from build123d import *

# Parameters (mm, degrees)
SKETCH1_W           = 25.4
SKETCH1_H           = 25.4
BOSS_EXTRUDE1_DEPTH = 228.6
FILLET1_R           = 1.5875
HOLE1_OUTLINE_R     = 2.5527
HOLE1_DEPTH         = 228.6
SKETCH7_W           = 6.5278
SKETCH7_H           = 2.2352
CUT_EXTRUDE2_DEPTH  = 228.6
FILLET4_R           = 0.396875
CIRPATTERN2_DEPTH   = 228.6


# Read off the part's stored shape, not the designer's step: Hole1, CirPattern2
with BuildPart() as part:
    # Sketch1 → Boss-Extrude1 (new body)
    with BuildSketch(Plane.XY):
        Rectangle(SKETCH1_W, SKETCH1_H)
    extrude(amount=BOSS_EXTRUDE1_DEPTH)

    # Fillet1
    fillet1_edges = [part.edges().sort_by_distance(p)[0] for p in [
        (12.7, -12.7, 114.3),
        (-12.7, -12.7, 114.3),
        (-12.7, 12.7, 114.3),
        (12.7, 12.7, 114.3),
    ]]
    fillet(fillet1_edges, radius=FILLET1_R)

    # Hole1 outline → Hole1 (cut)
    with BuildSketch(Plane.XY):
        with Locations((0, -0.048792482)):
            Circle(HOLE1_OUTLINE_R)
    extrude(amount=HOLE1_DEPTH, mode=Mode.SUBTRACT)

    # Sketch7 → Cut-Extrude2 (cut)
    with BuildSketch(Plane.XY.offset(228.6)):
        with Locations((0, 11.5824)):
            Rectangle(SKETCH7_W, SKETCH7_H)
        Polygon((-3.175, 4.5212), (-7.3025, 10.4648), (7.3025, 10.4648), (3.175, 4.5212), align=None)
    extrude(amount=-CUT_EXTRUDE2_DEPTH, mode=Mode.SUBTRACT)

    # Fillet4
    fillet4_edges = [part.edges().sort_by_distance(p)[0] for p in [
        (-3.2639, 10.4648, 114.3),
        (-3.2639, 12.7, 114.3),
        (3.2639, 12.7, 114.3),
        (3.2639, 10.4648, 114.3),
    ]]
    fillet(fillet4_edges, radius=FILLET4_R)

    # CirPattern2 outline → CirPattern2 (cut)
    with BuildSketch(Plane.XY):
        with BuildLine():
            ThreePointArc((-3.660775, -10.562384964), (-3.380141996, -10.67862696), (-3.2639, -10.959259964))
            Line((-3.2639, -10.959259964), (-3.2639, -12.7))
            Line((-3.2639, -12.7), (3.2639, -12.7))
            Line((3.2639, -12.7), (3.2639, -10.959259964))
            ThreePointArc((3.2639, -10.959259964), (3.380141996, -10.67862696), (3.660775, -10.562384964))
            Line((3.660775, -10.562384964), (7.3025, -10.562384964))
            Line((7.3025, -10.562384964), (3.175, -4.618784964))
            Line((3.175, -4.618784964), (-3.175, -4.618784964))
            Line((-3.175, -4.618784964), (-7.3025, -10.562384964))
            Line((-7.3025, -10.562384964), (-3.660775, -10.562384964))
        make_face()
        with BuildLine():
            Line((-12.7, -3.312692482), (-10.910467482, -3.312692482))
            ThreePointArc((-10.910467482, -3.312692482), (-10.629834478, -3.428934478), (-10.513592482, -3.709567482))
            Line((-10.513592482, -3.709567482), (-10.513592482, -7.351292482))
            Line((-10.513592482, -7.351292482), (-4.569992482, -3.223792482))
            Line((-4.569992482, -3.223792482), (-4.569992482, 3.126207518))
            Line((-4.569992482, 3.126207518), (-10.513592482, 7.253707518))
            Line((-10.513592482, 7.253707518), (-10.513592482, 3.611982518))
            ThreePointArc((-10.513592482, 3.611982518), (-10.629834478, 3.331349514), (-10.910467482, 3.215107518))
            Line((-10.910467482, 3.215107518), (-12.7, 3.215107518))
            Line((-12.7, 3.215107518), (-12.7, -3.312692482))
        make_face()
        with BuildLine():
            ThreePointArc((10.513592482, -3.709567482), (10.629834478, -3.428934478), (10.910467482, -3.312692482))
            Line((10.910467482, -3.312692482), (12.7, -3.312692482))
            Line((12.7, -3.312692482), (12.7, 3.215107518))
            Line((12.7, 3.215107518), (10.910467482, 3.215107518))
            ThreePointArc((10.910467482, 3.215107518), (10.629834478, 3.331349514), (10.513592482, 3.611982518))
            Line((10.513592482, 3.611982518), (10.513592482, 7.253707518))
            Line((10.513592482, 7.253707518), (4.569992482, 3.126207518))
            Line((4.569992482, 3.126207518), (4.569992482, -3.223792482))
            Line((4.569992482, -3.223792482), (10.513592482, -7.351292482))
            Line((10.513592482, -7.351292482), (10.513592482, -3.709567482))
        make_face()
    extrude(amount=CIRPATTERN2_DEPTH, mode=Mode.SUBTRACT)


solid = part.part
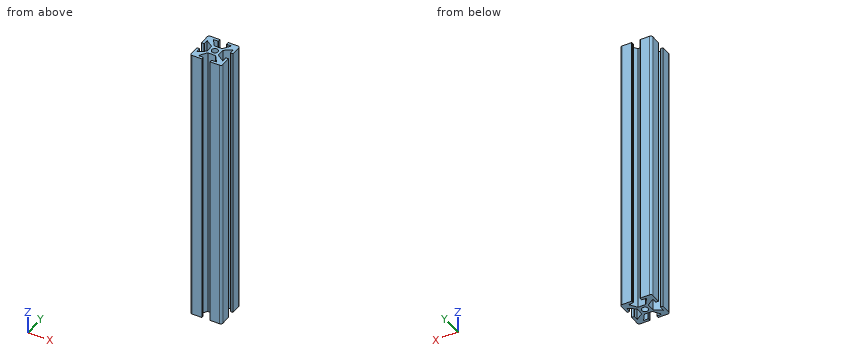
Work out the finished part from the listing and answer in its coordinate system (mm). Give positions to 0.01 mm unless a question says otherwise; leave off trailing zeros. Write each loop counter-clockwise with the first axis right and the second up, starting at its lowest first coordinate (ties: lowest second). Pieces come first, ordered by that corner, then holes.
Q1. Straight lines are drawn through the part: L1, parallel to Y at x = 11, z = 174; L2, parallel to Y at x = 0, z = 49.5; L3, parallel to X at y = 0, z = 47.5. For each, find the intervals that lie inside material, in ascending order.
Answer:
L1: y = -12.7 to -3.31, 3.22 to 12.7
L2: y = -4.62 to -2.6, 2.5 to 4.52
L3: x = -4.57 to -2.55, 2.55 to 4.57
Q2. The part is cut by section A-A on x = 0. Give the vertices of the cut face in (y, z).
Answer:
outline: (-4.62, 0) - (-2.6, 0) - (-2.6, 228.6) - (-4.62, 228.6) - close; (2.5, 0) - (4.52, 0) - (4.52, 228.6) - (2.5, 228.6) - close
Q3. Given pin 1 (0.5 mm diameter, centred on x = -11.5, z = 122.5, fed in from -Y); pin 2 (2 mm diameter, centred on y = -2, z = 59.5, fed in from +X); pin 3 (3 mm diameter, centred on x = 0, z = 74, fed in from -Y), each flat-ended and moving along its own axis, determine where each tip first touches the part or whether it passes through.
Answer:
pin 1: stops at y = -12.69
pin 2: stops at x = 4.57
pin 3: stops at y = -4.62
